Part model, mm, in its own coordinate system. A direction names the side the tool comes from. Give positions to 0.01 mm unless a question says otherwise; leave off trailing zeros. Write each loop counter-clockwise with the first axis right and the second up, starting at its lowest first coordinate (ties: lowest second). Pieces come first, ordered by that corner, then holes. Notation, with made-up numbers: M 49,10 L 94,10 A16 cw 94,19 Z; hole C -26.5,-13.75 d3. An arc over 180 degrees is marked long. Use a Markdown table: item, result. Add a question column.
Autodesk Inventor part; units mm, degrees
ref_plane "YZ Plane" through (0, 0, 0) normal (1, 0, 0) x (0, 1, 0)
ref_plane "XZ Plane" through (0, 0, 0) normal (0, 1, 0) x (-1, 0, 0)
ref_plane "XY Plane" through (0, 0, 0) normal (0, 0, 1) x (1, 0, 0)
sketch "Sketch1" plane through (0, 0, 0) normal (0, 1, 0) x (-1, 0, 0)
  line L0 (-250, 250) -> (250, 250)
  line L1 (250, 250) -> (250, -250)
  line L2 (250, -250) -> (-250, -250)
  line L3 (-250, -250) -> (-250, 250)
  line L4 (-250, 250) -> (250, -250) construction
  line L5 (250, 250) -> (-250, -250) construction
  line L6 (-12.4264, 42.4417) -> (30, 0.0153)
  line L7 (30, 0.0153) -> (-12.4264, -42.4112)
  line L8 (-12.4264, -42.4112) -> (-54.8528, 0.0153)
  line L9 (-54.8528, 0.0153) -> (-12.4264, 42.4417)
  point P0 (0, 0)
  dimension "d0" = 500
  dimension "d1" = 60
  dimension "d2" = 30
  dimension "d3" = 54.8528
extrude "Extrusion1" add sketch "Sketch1" along normal blind 10
properties part number "wer"
1. Tool access for faces 1 (the flat face through (-8.49, 4.93, 21.525)), 2 (the flat face through (59, 10, 4)): list every direction of +Z, -Z, +X, -X, +Y, -Y with a clear straight run to the whole face (end or side of a thin tool).
2. Drill centre lines: probe 1 along X at (y, z) = (3.25, 13); probe 2 along X at (y, z) = (3, -32). Where is each one in solid material? Low to high. Write a range as [from, to].
3. Cut at A-A (x = 31.5). Write the cut outline in (y, z), then the cut area to 3 significant figures.
4. Mould opens along Z. For faces 3 (the flat face through (-9.084, 4.93, -20.901)), 4 (the flat face through (59, 0, 4)) say: released by +Z, released by -Z, zero draft, split by the parting line, or undercut.
A:
| question | item | result |
|---|---|---|
| 1 | face 1 | +Y, -Y |
| 1 | face 2 | +Z, -Z, +X, -X, +Y |
| 2 | probe 1 | x = [-250, -17.02], [41.87, 250] |
| 2 | probe 2 | x = [-250, 2.02], [22.84, 250] |
| 3 | outline | M 0,-250 L 10,-250 L 10,-23.34 L 0,-23.34 Z; M 0,23.37 L 10,23.37 L 10,250 L 0,250 Z |
| 3 | area | 4,530 mm² |
| 4 | face 3 | undercut |
| 4 | face 4 | zero draft |
